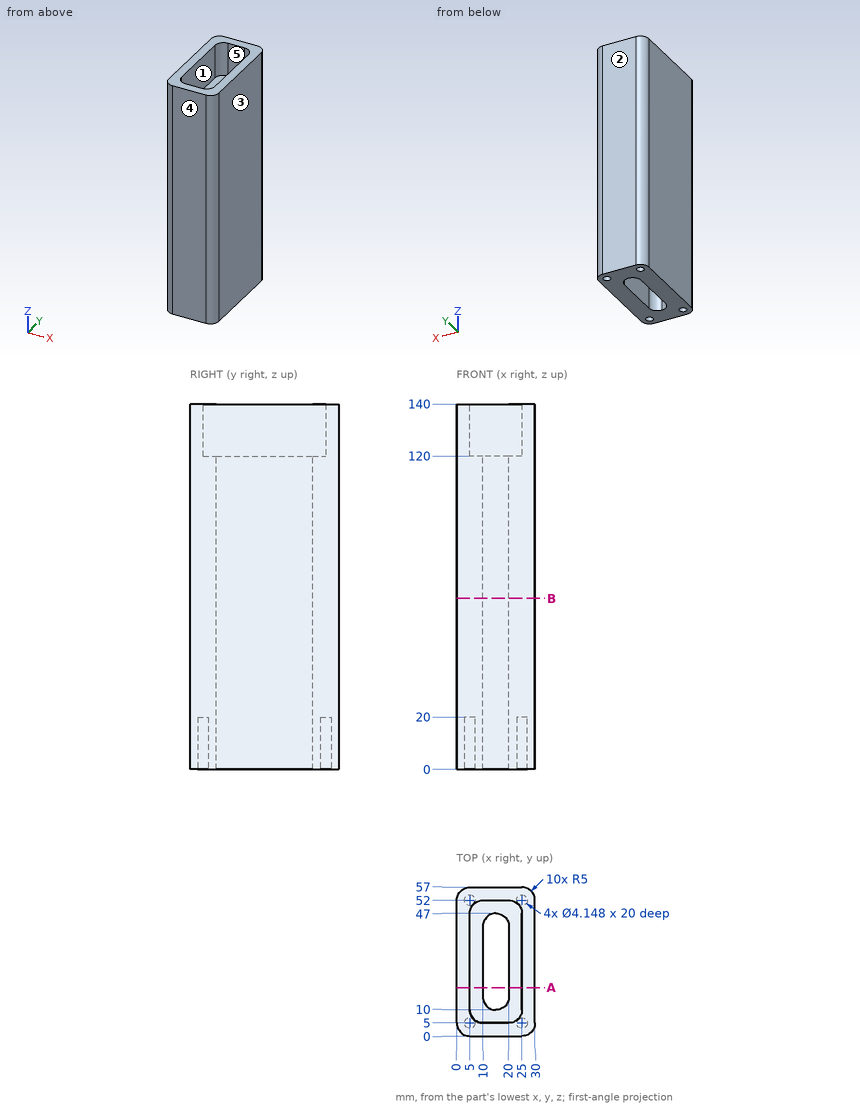
Verification items for this drawing (mm, ordinates from the low corner). A direction names the side the tool comes from. Coordinates: 2 decimals unless noted, no trailing zeros. Write each loop counter-clockwise with the first axis right and the second up, starting at its lowest first coordinate (ties: lowest second). Pieces come first, ordered by that corner, then holes. Notation, with made-up numbers: M 31,61 L 84,61 A28 cw 84,81 Z; hole C 24,-14.75 d4. An arc over 180 degrees is marked long. Answer as a JSON object with one key per item and string values.
1. Tool access check on the marked faces 1 and 2. Record the directions out of +Z, -Z, +X, -X, +Y, -Y that give a thin tool (end or side, any length) a straight path to the whole face; none if there is none.
Answers below:
{"face 1": "+Z", "face 2": "+Z, -Z, +X, -X, +Y"}
2. Section check B-B, the plane z = 65.5. Enter the section's corners in (x, y), plus the area to 3 significant figures.
Answers below:
{"outline": "M 0,5 A5 ccw 5,0 L 25,0 A5 ccw 30,5 L 30,52 A5 ccw 25,57 L 5,57 A5 ccw 0,52 Z; hole M 10,15 A5 ccw 20,15 L 20,42 A5 ccw 10,42 Z", "area": "1,340 mm²"}
3. Go/stop test with flat-tipped pins: pin 1 Ø2 at (x, y) = (5.5, 51.5) entering from -Z; pin 2 Ø8 at (x, y) = (17.5, 24.5) entering from +Z; pin 3 Ø1.5 at (x, z) = (4, 16) entering from +Y. Record where each tip stops, or that it passes through.
Answers below:
{"pin 1": "stops at z = 20", "pin 2": "stops at z = 120", "pin 3": "stops at y = 56.99"}
4. Section check A-A, the plane y = 18.5. Enter the section's corners in (x, z).
Answers below:
{"outline": "M 0,0 L 10,0 L 10,120 L 5,120 L 5,140 L 0,140 Z; M 20,0 L 30,0 L 30,140 L 25,140 L 25,120 L 20,120 Z"}
5. Scan lines: L1, parallel to X at y = 5, z = 10; L2, parallel to X at y = 21, z = 15.5; L3, parallel to Z at x = 15, y = 49. Record each from-to range of solid material in increasing order.
Answers below:
{"L1": "x = 0 to 2.93, 7.07 to 22.93, 27.07 to 30", "L2": "x = 0 to 10, 20 to 30", "L3": "z = 0 to 120"}
6. Draft check along X on the marked faces 3, 4 and 5. Enter one of: released by +X, released by -X, zero draft, split by the parting line, or undercut.
Answers below:
{"face 3": "released by +X", "face 4": "zero draft", "face 5": "undercut"}
